```python
from build123d import *

# Parameters (mm, degrees)
F1_DEPTH     = 31
F3_DEPTH     = 26
F5_DEPTH     = 10
F6_T1_DEPTH  = 67
F6_T3_DEPTH  = 67
F6_T6_ANGLE  = 90
F6_T8_ANGLE  = 90
F6_T10_ANGLE = 90
F6_T12_ANGLE = 90
F6_T13_DEPTH = 67
F6_T15_DEPTH = 67
F6_T17_DEPTH = 3.5
F6_T19_DEPTH = 3.5
F6_T21_DEPTH = 2
F6_T23_DEPTH = 16
F6_T26_ANGLE = 90
F6_T28_ANGLE = 90
F6_T30_ANGLE = 90
F6_T32_ANGLE = 90
F6_T34_ANGLE = 90
F6_T36_ANGLE = 90
F6_T38_ANGLE = 90
F6_T40_ANGLE = 90
F6_T42_ANGLE = 90
F6_T44_ANGLE = 90
F6_T46_ANGLE = 90
F6_T48_ANGLE = 90
F6_T50_ANGLE = 90
F6_T52_ANGLE = 90
F6_T54_ANGLE = 90
F6_T56_ANGLE = 90
F6_T58_ANGLE = 90
F6_T60_ANGLE = 90
F6_T62_ANGLE = 90
F6_T64_ANGLE = 90


# Not quite as in the source:
# - a fillet or chamfer that OpenCascade refuses, or shapes differently, is made with other operations: its cross-section is extruded or revolved along the edge and cut away or added


with BuildPart() as f1:
    # F0 (on Top) → F1 (new body)
    with BuildSketch(Plane.XY):
        with BuildLine():
            Line((55.5, -33.5), (55.5, 33.5))
            ThreePointArc((55.5, 33.5), (49.0563491861, 49.0563491861), (33.5, 55.5))
            Line((33.5, 55.5), (-33.5, 55.5))
            ThreePointArc((-33.5, 55.5), (-49.0563491861, 49.0563491861), (-55.5, 33.5))
            Line((-55.5, 33.5), (-55.5, -33.5))
            ThreePointArc((-55.5, -33.5), (-49.0563491861, -49.0563491861), (-33.5, -55.5))
            Line((-33.5, -55.5), (33.5, -55.5))
            ThreePointArc((33.5, -55.5), (49.0563491861, -49.0563491861), (55.5, -33.5))
        make_face()
    extrude(amount=F1_DEPTH)

    # F2 (on face) → F3 (cut, through all)
    with BuildSketch(Plane.XY.offset(31)):
        with BuildLine():
            Line((33.5, 45.5), (-33.5, 45.5))
            ThreePointArc((-33.5, 45.5), (-41.9852813742, 41.9852813742), (-45.5, 33.5))
            Line((-45.5, 33.5), (-45.5, -33.5))
            ThreePointArc((-45.5, -33.5), (-41.9852813742, -41.9852813742), (-33.5, -45.5))
            Line((-33.5, -45.5), (33.5, -45.5))
            ThreePointArc((33.5, -45.5), (41.9852813742, -41.9852813742), (45.5, -33.5))
            Line((45.5, -33.5), (45.5, 33.5))
            ThreePointArc((45.5, 33.5), (41.9852813742, 41.9852813742), (33.5, 45.5))
        make_face()
    extrude(amount=-F3_DEPTH, mode=Mode.SUBTRACT)

    # F4 (on face) → F5 (cut, through all)
    with BuildSketch(Plane.XZ.offset(55.5)):
        with BuildLine():
            ThreePointArc((-30, 31), (-21.5147186258, 27.4852813742), (-18, 19))
            Line((-18, 19), (-18, 17))
            ThreePointArc((-18, 17), (-15.0710678119, 9.9289321881), (-8, 7))
            Line((-8, 7), (8, 7))
            ThreePointArc((8, 7), (15.0710678119, 9.9289321881), (18, 17))
            Line((18, 17), (18, 19))
            ThreePointArc((18, 19), (21.5147186258, 27.4852813742), (30, 31))
            Line((30, 31), (-30, 31))
        make_face()
    extrude(amount=-F5_DEPTH, mode=Mode.SUBTRACT)

    # F6: chamfer of 2 x 1 on 48 edges, made by hand

    # F6_s2 → F6_t1 (join)
    with BuildSketch(Plane.XZ.offset(-33.5)):
        Polygon((-45.5, 6), (-43.5, 5), (-45.5, 5), align=None)
        Polygon((45.5, 6), (43.5, 5), (45.5, 5), align=None)
    extrude(amount=F6_T1_DEPTH)

    # F6_s4 → F6_t3 (join)
    with BuildSketch(Plane.YZ.offset(-33.5)):
        Polygon((-45.5, 6), (-43.5, 5), (-45.5, 5), align=None)
        Polygon((45.5, 6), (43.5, 5), (45.5, 5), align=None)
    extrude(amount=F6_T3_DEPTH)

    # F6_s5 → F6_t6 (revolve)
    with BuildSketch(Plane.YZ.offset(33.5)):
        Polygon((-45.5, 6), (-43.5, 5), (-45.5, 5), align=None)
    revolve(axis=Axis((33.5, -33.5, 5), (0, 0, 1)), revolution_arc=F6_T6_ANGLE)

    # F6_s7 → F6_t8 (revolve)
    with BuildSketch(Plane.XZ.offset(-33.5)):
        Polygon((45.5, 6), (43.5, 5), (45.5, 5), align=None)
    revolve(axis=Axis((33.5, 33.5, 5), (0, 0, 1)), revolution_arc=F6_T8_ANGLE)

    # F6_s9 → F6_t10 (revolve)
    with BuildSketch(Plane.YZ.offset(-33.5)):
        Polygon((45.5, 6), (43.5, 5), (45.5, 5), align=None)
    revolve(axis=Axis((-33.5, 33.5, 5), (0, 0, 1)), revolution_arc=F6_T10_ANGLE)

    # F6_s11 → F6_t12 (revolve)
    with BuildSketch(Plane.XZ.offset(33.5)):
        Polygon((-45.5, 6), (-43.5, 5), (-45.5, 5), align=None)
    revolve(axis=Axis((-33.5, -33.5, 5), (0, 0, 1)), revolution_arc=F6_T12_ANGLE)

    # F6_s14 → F6_t13 (cut)
    with BuildSketch(Plane.YZ.offset(-33.5)):
        Polygon((47.5, 31), (45.5, 30), (45.5, 31), align=None)
        Polygon((53.5, 31), (55.5, 30), (55.5, 31), align=None)
        Polygon((-54.5, 0), (-55.5, 2), (-55.5, 0), align=None)
        Polygon((54.5, 0), (55.5, 2), (55.5, 0), align=None)
    extrude(amount=F6_T13_DEPTH, mode=Mode.SUBTRACT)

    # F6_s16 → F6_t15 (cut)
    with BuildSketch(Plane.XZ.offset(-33.5)):
        Polygon((55.5, 2), (54.5, 0), (55.5, 0), align=None)
        Polygon((55.5, 30), (53.5, 31), (55.5, 31), align=None)
        Polygon((-54.5, 0), (-55.5, 2), (-55.5, 0), align=None)
        Polygon((47.5, 31), (45.5, 30), (45.5, 31), align=None)
        Polygon((-47.5, 31), (-45.5, 30), (-45.5, 31), align=None)
        Polygon((-53.5, 31), (-55.5, 30), (-55.5, 31), align=None)
    extrude(amount=F6_T15_DEPTH, mode=Mode.SUBTRACT)

    # F6_s18 → F6_t17 (cut)
    with BuildSketch(Plane.YZ.offset(30)):
        Polygon((-53.5, 31), (-55.5, 30), (-55.5, 31), align=None)
        Polygon((-47.5, 31), (-45.5, 30), (-45.5, 31), align=None)
    extrude(amount=F6_T17_DEPTH, mode=Mode.SUBTRACT)

    # F6_s20 → F6_t19 (cut)
    with BuildSketch(Plane.YZ.offset(-33.5)):
        Polygon((-47.5, 31), (-45.5, 30), (-45.5, 31), align=None)
        Polygon((-53.5, 31), (-55.5, 30), (-55.5, 31), align=None)
    extrude(amount=F6_T19_DEPTH, mode=Mode.SUBTRACT)

    # F6_s22 → F6_t21 (cut)
    with BuildSketch(Plane.XY.offset(17)):
        Polygon((19, -55.5), (18, -53.5), (18, -55.5), align=None)
        Polygon((-19, -55.5), (-18, -53.5), (-18, -55.5), align=None)
        Polygon((-19, -45.5), (-18, -47.5), (-18, -45.5), align=None)
        Polygon((19, -45.5), (18, -47.5), (18, -45.5), align=None)
    extrude(amount=F6_T21_DEPTH, mode=Mode.SUBTRACT)

    # F6_s24 → F6_t23 (cut)
    with BuildSketch(Plane.YZ.offset(-8)):
        Polygon((-55.5, 6), (-53.5, 7), (-55.5, 7), align=None)
        Polygon((-45.5, 6), (-47.5, 7), (-45.5, 7), align=None)
    extrude(amount=F6_T23_DEPTH, mode=Mode.SUBTRACT)

    # F6_s25 → F6_t26 (revolve, cut)
    with BuildSketch(Plane.YZ.offset(33.5)):
        Polygon((-55.5, 2), (-54.5, 0), (-55.5, 0), align=None)
    revolve(axis=Axis((33.5, -33.5, 0), (0, 0, 1)), revolution_arc=F6_T26_ANGLE, mode=Mode.SUBTRACT)

    # F6_s27 → F6_t28 (revolve, cut)
    with BuildSketch(Plane.YZ.offset(33.5)):
        Polygon((-55.5, 30), (-53.5, 31), (-55.5, 31), align=None)
    revolve(axis=Axis((33.5, -33.5, 31), (0, 0, 1)), revolution_arc=F6_T28_ANGLE, mode=Mode.SUBTRACT)

    # F6_s29 → F6_t30 (revolve, cut)
    with BuildSketch(Plane.XZ.offset(-33.5)):
        Polygon((55.5, 2), (54.5, 0), (55.5, 0), align=None)
    revolve(axis=Axis((33.5, 33.5, 0), (0, 0, 1)), revolution_arc=F6_T30_ANGLE, mode=Mode.SUBTRACT)

    # F6_s31 → F6_t32 (revolve, cut)
    with BuildSketch(Plane.XZ.offset(-33.5)):
        Polygon((55.5, 30), (53.5, 31), (55.5, 31), align=None)
    revolve(axis=Axis((33.5, 33.5, 31), (0, 0, 1)), revolution_arc=F6_T32_ANGLE, mode=Mode.SUBTRACT)

    # F6_s33 → F6_t34 (revolve, cut)
    with BuildSketch(Plane.YZ.offset(-33.5)):
        Polygon((54.5, 0), (55.5, 2), (55.5, 0), align=None)
    revolve(axis=Axis((-33.5, 33.5, 0), (0, 0, 1)), revolution_arc=F6_T34_ANGLE, mode=Mode.SUBTRACT)

    # F6_s35 → F6_t36 (revolve, cut)
    with BuildSketch(Plane.XZ.offset(33.5)):
        Polygon((-54.5, 0), (-55.5, 2), (-55.5, 0), align=None)
    revolve(axis=Axis((-33.5, -33.5, 0), (0, 0, 1)), revolution_arc=F6_T36_ANGLE, mode=Mode.SUBTRACT)

    # F6_s37 → F6_t38 (revolve, cut)
    with BuildSketch(Plane.YZ.offset(33.5)):
        Polygon((-47.5, 31), (-45.5, 30), (-45.5, 31), align=None)
    revolve(axis=Axis((33.5, -33.5, 31), (0, 0, 1)), revolution_arc=F6_T38_ANGLE, mode=Mode.SUBTRACT)

    # F6_s39 → F6_t40 (revolve, cut)
    with BuildSketch(Plane.XZ.offset(-33.5)):
        Polygon((47.5, 31), (45.5, 30), (45.5, 31), align=None)
    revolve(axis=Axis((33.5, 33.5, 31), (0, 0, 1)), revolution_arc=F6_T40_ANGLE, mode=Mode.SUBTRACT)

    # F6_s41 → F6_t42 (revolve, cut)
    with BuildSketch(Plane.YZ.offset(-33.5)):
        Polygon((47.5, 31), (45.5, 30), (45.5, 31), align=None)
    revolve(axis=Axis((-33.5, 33.5, 31), (0, 0, 1)), revolution_arc=F6_T42_ANGLE, mode=Mode.SUBTRACT)

    # F6_s43 → F6_t44 (revolve, cut)
    with BuildSketch(Plane.XZ.offset(33.5)):
        Polygon((-47.5, 31), (-45.5, 30), (-45.5, 31), align=None)
    revolve(axis=Axis((-33.5, -33.5, 31), (0, 0, 1)), revolution_arc=F6_T44_ANGLE, mode=Mode.SUBTRACT)

    # F6_s45 → F6_t46 (revolve, cut)
    with BuildSketch(Plane.XZ.offset(33.5)):
        Polygon((-53.5, 31), (-55.5, 30), (-55.5, 31), align=None)
    revolve(axis=Axis((-33.5, -33.5, 31), (0, 0, 1)), revolution_arc=F6_T46_ANGLE, mode=Mode.SUBTRACT)

    # F6_s47 → F6_t48 (revolve, cut)
    with BuildSketch(Plane.YZ.offset(-33.5)):
        Polygon((53.5, 31), (55.5, 30), (55.5, 31), align=None)
    revolve(axis=Axis((-33.5, 33.5, 31), (0, 0, 1)), revolution_arc=F6_T48_ANGLE, mode=Mode.SUBTRACT)

    # F6_s49 → F6_t50 (revolve, cut)
    with BuildSketch(Plane.XY.offset(19)):
        Polygon((19, -55.5), (18, -53.5), (18, -55.5), align=None)
    revolve(axis=Axis((30, -55.5, 19), (0, 1, 0)), revolution_arc=F6_T50_ANGLE, mode=Mode.SUBTRACT)

    # F6_s51 → F6_t52 (revolve, cut)
    with BuildSketch(Plane.YZ.offset(8)):
        Polygon((-55.5, 6), (-53.5, 7), (-55.5, 7), align=None)
    revolve(axis=Axis((8, -55.5, 17), (0, -1, 0)), revolution_arc=F6_T52_ANGLE, mode=Mode.SUBTRACT)

    # F6_s53 → F6_t54 (revolve, cut)
    with BuildSketch(Plane.XY.offset(17)):
        Polygon((-19, -55.5), (-18, -53.5), (-18, -55.5), align=None)
    revolve(axis=Axis((-8, -55.5, 17), (0, -1, 0)), revolution_arc=F6_T54_ANGLE, mode=Mode.SUBTRACT)

    # F6_s55 → F6_t56 (revolve, cut)
    with BuildSketch(Plane.YZ.offset(-30)):
        Polygon((-55.5, 30), (-53.5, 31), (-55.5, 31), align=None)
    revolve(axis=Axis((-30, -55.5, 19), (0, 1, 0)), revolution_arc=F6_T56_ANGLE, mode=Mode.SUBTRACT)

    # F6_s57 → F6_t58 (revolve, cut)
    with BuildSketch(Plane.XY.offset(19)):
        Polygon((18, -47.5), (19, -45.5), (18, -45.5), align=None)
    revolve(axis=Axis((30, -45.5, 19), (0, 1, 0)), revolution_arc=F6_T58_ANGLE, mode=Mode.SUBTRACT)

    # F6_s59 → F6_t60 (revolve, cut)
    with BuildSketch(Plane.YZ.offset(-30)):
        Polygon((-45.5, 30), (-47.5, 31), (-45.5, 31), align=None)
    revolve(axis=Axis((-30, -45.5, 19), (0, 1, 0)), revolution_arc=F6_T60_ANGLE, mode=Mode.SUBTRACT)

    # F6_s61 → F6_t62 (revolve, cut)
    with BuildSketch(Plane.XY.offset(17)):
        Polygon((-19, -45.5), (-18, -47.5), (-18, -45.5), align=None)
    revolve(axis=Axis((-8, -45.5, 17), (0, -1, 0)), revolution_arc=F6_T62_ANGLE, mode=Mode.SUBTRACT)

    # F6_s63 → F6_t64 (revolve, cut)
    with BuildSketch(Plane.YZ.offset(8)):
        Polygon((-45.5, 6), (-47.5, 7), (-45.5, 7), align=None)
    revolve(axis=Axis((8, -45.5, 17), (0, -1, 0)), revolution_arc=F6_T64_ANGLE, mode=Mode.SUBTRACT)


solid = f1.part
```
Verification items for the finished model (mm, model axes). A direction names the side the tool comes from. Round coordinates to 2 decimals unless told otherwise and drop trailing zeros. Write each loop counter-clockwise with the first axis right and the second up, starting at its lowest first coordinate (ties: lowest second). Pieces come first, ordered by that corner, then holes.
1. Section check A-A on y = 7. Enter the section's corners in (x, z).
2. Access from +Z, -Z, +X, -X, +Y, -Y to the whole of each face (thin tool, end or side, straight path). Record for faces 1 (the conical face through (40.72, -40.88, 5.16)), 2 (the cylindrical face through (-15.15, -50.54, 10.01)), 3 (the flat face through (-55.5, 0, 16)).
3. Scan lines: L1, parallel to X at y = -31, z = 19; L2, parallel to Z at x = -7.5, y = 9.5. Record each from-to range of solid material in increasing order.
4. Draft check along Y on faces 4 (the conical face through (15.18, -46.96, 9.66)), 5 (the conical face through (48.03, 47.71, 30.84)), 6 (the flat face through (0, -51, 7)). Enter one of: +Y half, -Y half, draft (parallel to the pull), parting line (faces both ways), or undercut.
5. Gauge pin test, flat ends, axial feed: P1, Ø1, axis at y = -51.5, z = 17.5, coming from the -X side; P2, Ø1, axis at y = 42, z = 22, coming from the +X side; P3, Ø6, axis at x = 38.5, z = 17, coming from the -Y side. Record the tip position at first contact, or that the pin passes through.
Answer:
1. outline: (-55.5, 2) - (-54.5, 0) - (54.5, 0) - (55.5, 2) - (55.5, 30) - (53.5, 31) - (47.5, 31) - (45.5, 30) - (45.5, 6) - (43.5, 5) - (-43.5, 5) - (-45.5, 6) - (-45.5, 30) - (-47.5, 31) - (-53.5, 31) - (-55.5, 30) - close
2. face 1: +Z
2. face 2: +Z, -Y
2. face 3: +Z, -Z, -X, +Y, -Y
3. L1: x = -55.5 to -45.5, 45.5 to 55.5
3. L2: z = 0 to 5
4. face 4: undercut
4. face 5: +Y half
4. face 6: draft
5. P1: stops at x = -46.83
5. P2: stops at x = 53.99
5. P3: stops at y = -55.41
